Geometry check sheet. Reference: drawing and pictorial views, mm from the part's lowest x, y, z. Coordinates: 2 decimals unless noted, no trailing zeros. Loops run counter-clockwise (first coordinate to the right, second up) from the corner with the lowest first, then second, coordinate; pieces in that order, holes last.
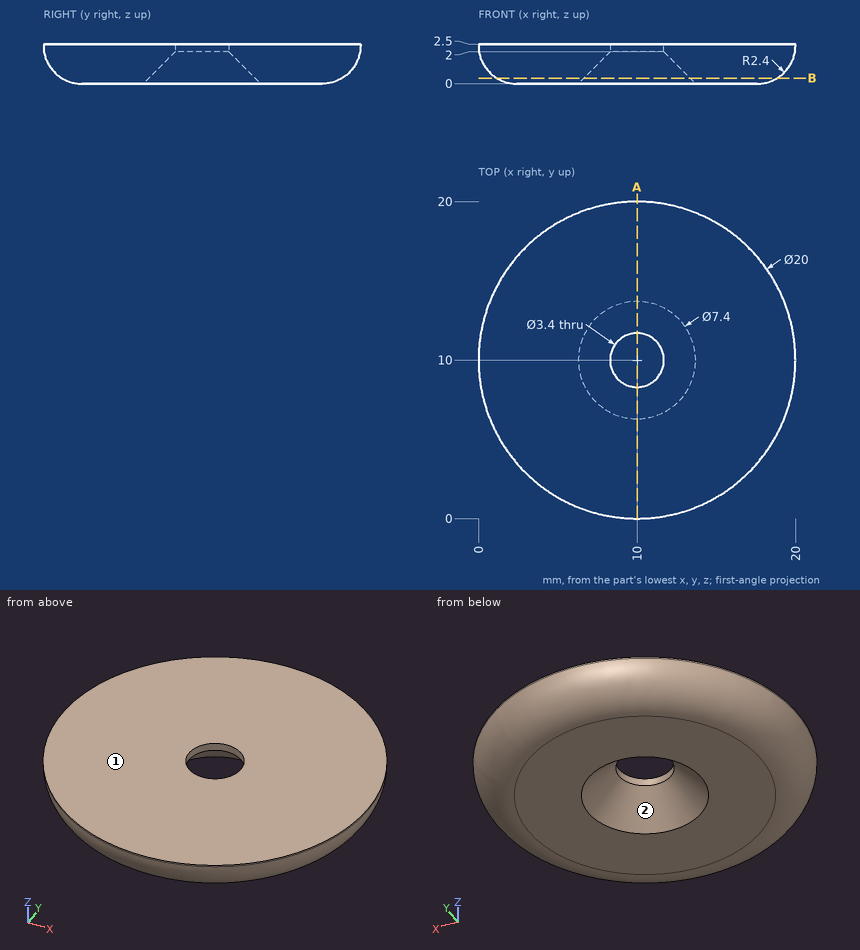
1) Material ranges on probe 1 along Y at (x, z) = (10, 2.35); probe 2 along Y at (x, z) = (11.5, 1.35); probe 3 along X at (y, z) = (17.75, 1.4), recorded low to high.
Data:
probe 1: y = 0 to 8.3, 11.7 to 20
probe 2: y = 0.36 to 8.19, 11.81 to 19.64
probe 3: x = 4.03 to 15.97
2) Mould release check, pull along Y, two halves, no side actions. Record for the marked faces 1 and 2: +Y half, -Y half, draft (parallel to the pull), parting line (faces both ways), or undercut.
Data:
face 1: draft
face 2: undercut
3) Section check A-A on x = 10. Record the cut outline in (y, z).
Data:
outline: (0, 2.4) arc R2.4 ccw to (2.4, 0) - (6.3, 0) - (8.3, 2) - (8.3, 2.5) - (0, 2.5) - close; (11.7, 2) - (13.7, 0) - (17.6, 0) arc R2.4 ccw to (20, 2.4) - (20, 2.5) - (11.7, 2.5) - close
4) Section check B-B on z = 0.35. Record the cut outline in (x, y), and give its area (3 significant figures).
Data:
outline: circle Ø17.7 at (10, 10); hole circle Ø6.7 at (10, 10)
area: 211 mm2
5) Depth check by flat-ended pin: pin 1 (2.5 mm diameter, centred on x = 10, y = 10, fed in from -Z); pin 2 (1.5 mm diameter, centred on x = 16.5, y = 15, fed in from -Z); pin 3 (1 mm diameter, centred on y = 11, z = 1, fed in from +X). Enter the tip coordinate at first touch or a pass-through.
Data:
pin 1: passes through
pin 2: stops at z = 0
pin 3: stops at x = 19.78
